Verification items for this drawing (mm, ordinates from the low corner). A direction names the side the tool comes from. Give positions to 0.01 mm unless a question says otherwise; leave off trailing zeros. Loops run counter-clockwise (first coordinate to the right, second up) from the corner with the lowest first, then second, coordinate; pieces in that order, holes last. Notation, with made-up numbers: (69.5, 33) -> (126.5, 33) arc R33 ccw to (126.5, 67) -> close; hole circle Ø1 at (44, 44.5). An arc over 180 degrees is marked (long way). Answer in a Markdown table with one row per item. Add a question column.
Q1. Material ranges on probe 1 along Y at (x, z) = (50, 25.65); probe 2 along Y at (x, z) = (47.5, 24.75); probe 3 along Z at (x, y) = (48, 48), recorded low to high.
Q2. Section check C-C on x = 50. Enter the section's corners in (y, z), and give its area (3 significant figures).
Q3. Set-up check for the marked faces 1 and 2: record each of +Z, -Z, +X, -X, +Y, -Y from which the full face is reachable in a straight line by a thin tool's end or side.
Q4. Section check B-B on z = 8. Enter the section's corners in (x, y), and give its area (3 significant figures).
Q5. Section check A-A on y = 42. Enter the section's corners in (x, z).
Q6. Section check D-D on x = 16. Enter the section's corners in (y, z).
Q7. Gauge pin test, flat ends, axial feed: P1, Ø6.5, axis at x = 10, y = 22, coming from the +Z side; P2, Ø3, axis at x = 16, y = 16, coming from the -Z side; P3, Ø3, axis at x = 11.5, z = 13.5, coming from the +Y side. Record the tip position at first contact, or that the pin passes through.
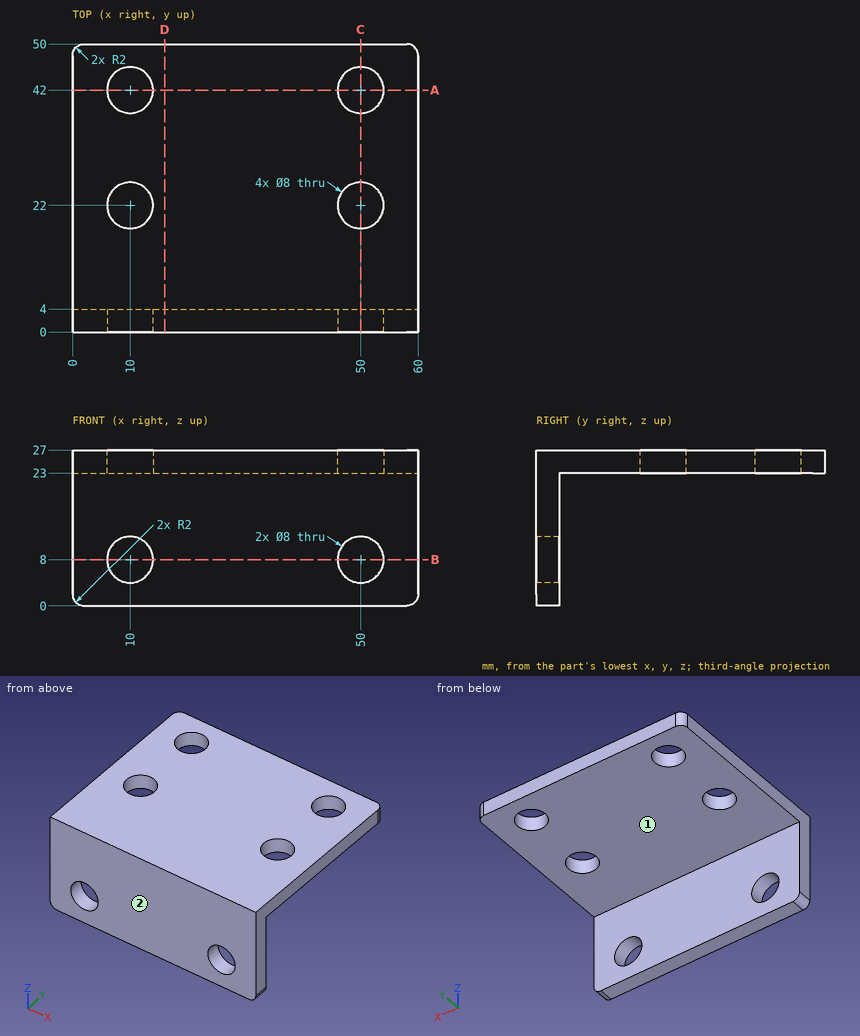
Taken from the geometry:
| question | item | result |
|---|---|---|
| 1 | probe 1 | y = 0 to 18, 26 to 38, 46 to 50 |
| 1 | probe 2 | y = 0 to 18.88, 25.12 to 38.88, 45.12 to 50 |
| 1 | probe 3 | z = 23 to 27 |
| 2 | outline | (0, 0) -> (4, 0) -> (4, 4) -> (0, 4) -> close; (0, 12) -> (4, 12) -> (4, 23) -> (18, 23) -> (18, 27) -> (0, 27) -> close; (26, 23) -> (38, 23) -> (38, 27) -> (26, 27) -> close; (46, 23) -> (50, 23) -> (50, 27) -> (46, 27) -> close |
| 2 | area | 196 mm² |
| 3 | face 1 | -Z, +X, -X, +Y |
| 3 | face 2 | +Z, -Z, +X, -X, -Y |
| 4 | outline | (0, 0) -> (6, 0) -> (6, 4) -> (0, 4) -> close; (14, 0) -> (46, 0) -> (46, 4) -> (14, 4) -> close; (54, 0) -> (60, 0) -> (60, 4) -> (54, 4) -> close |
| 4 | area | 176 mm² |
| 5 | outline | (0, 23) -> (6, 23) -> (6, 27) -> (0, 27) -> close; (14, 23) -> (46, 23) -> (46, 27) -> (14, 27) -> close; (54, 23) -> (60, 23) -> (60, 27) -> (54, 27) -> close |
| 6 | outline | (0, 0) -> (4, 0) -> (4, 23) -> (50, 23) -> (50, 27) -> (0, 27) -> close |
| 7 | P1 | passes through |
| 7 | P2 | stops at z = 23 |
| 7 | P3 | stops at y = 4 |
